```python
from build123d import *

# Parameters (mm, degrees)
EXTRUDE_1_DEPTH             = 8
CUT_EXTRUDE_1_DEPTH         = 5
HOLE_WIZARD_M51_D           = 5.2
HOLE_WIZARD_M51_DEPTH       = 4.2
HOLE_WIZARD_M51_CBORE_D     = 12
HOLE_WIZARD_M51_CBORE_DEPTH = 3
FILLET_1_R                  = 1


with BuildPart() as part:
    # Эскиз1 → Бобышка-Вытянуть1 (new body, symmetric)
    with BuildSketch(Plane.XY):
        Polygon((11, 0), (-11, 0), (-11, 9.2), (-6.75, 9.2), (-6.75, 5.7), (-5.25, 4.2), (5.25, 4.2), (6.75, 5.7), (6.75, 9.2), (11, 9.2), align=None)
    extrude(amount=EXTRUDE_1_DEPTH, both=True)

    # Эскиз2 → Вырез-Вытянуть1 (cut, symmetric)
    with BuildSketch(Plane.XY):
        Polygon((-11, 7.7), (-6.75, 7.7), (-6.75, 5.7), (-5.25, 4.2), (-6.5, 4.2), (-6.5, 0), (-11, 0), align=None)
    cut_extrude_1 = extrude(amount=CUT_EXTRUDE_1_DEPTH, both=True, mode=Mode.SUBTRACT)

    # Зеркальное отражение1: Вырез-Вытянуть1 across plane
    add(cut_extrude_1.mirror(Plane(origin=(0, 0, 0), x_dir=(0, 0, 1), z_dir=(1, 0, 0))), mode=Mode.SUBTRACT)

    # Цековка для  болта с шестигранной головкой M51
    with Locations(Plane(origin=(0, 4.2, 0), x_dir=(1, 0, 0), z_dir=(0, 1, 0))):
        with Locations((0, 0)):
            CounterBoreHole(HOLE_WIZARD_M51_D / 2, HOLE_WIZARD_M51_CBORE_D / 2, HOLE_WIZARD_M51_CBORE_DEPTH, depth=HOLE_WIZARD_M51_DEPTH)

    # Скругление1
    fillet_1_edges = [part.edges().sort_by_distance(p)[0] for p in [
        (11, 4.6, 8),
        (11, 4.6, -8),
        (-11, 4.6, -8),
        (-11, 4.6, 8),
    ]]
    fillet(fillet_1_edges, radius=FILLET_1_R)


solid = part.part
```
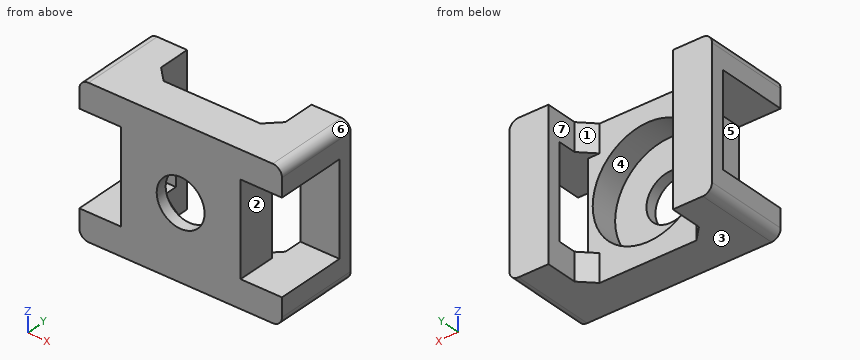
The listing builds one solid part. Answer for the finished solid, in the listing's coordinates (mm). Face numbers are marked on the shaded views. A direction names the side the tool comes from. Round coordinates to 2 decimals unless told otherwise and drop trailing zeros. Order: outer loops, then holes, each group sorted by start corner. A loop starts at its lowest first (then second) coordinate and runs counter-clockwise, first axis right, second up. Notation, with made-up numbers: (46, 57.25) - (88, 57.25) arc R7 cw to (88, 62.25) - close; hole circle Ø8 at (-12, -27.75). An arc over 180 degrees is marked (long way). Put each result on its own line as item: value. Start each with the question number.
(1) Given P1, Ø6, axis at x = 0, z = 0, coming from the +Y side; P2, Ø4, axis at x = -2, z = 3.5, coming from the +Y side; P3, Ø4.5, axis at y = 2, z = 2, coming from the -X side, each flat-ended and moving along its own axis, determine where each tip first touches the part or whether it passes through.
(2) Determine the mould class of the marked faces 1, 2 and 3 for opening direction X: released by +X, released by -X, zero draft, split by the parting line, or undercut.
(3) Find section D-D (y = 6.5). Give the vertices of the cut face in (x, z).
(4) Find section A-A (z = 0). Give the vertices of the cut face in (x, y).
(5) Find section B-B (y = 1.75). Give the vertices of the cut face in (x, z).
(6) Straight lines are drawn through the part: probe 1 along Z at (x, y) = (0, 0.3); probe 2 along Z at (x, y) = (0, 2.55); probe 3 along Y at (x, z) = (1.25, -3). For each, find the intervals that lie inside material, in ascending order. Write a range as from..to.
(7) For the marked faces 4, 5, 6 and 7, determine the directions among +Z, -Z, +X, -X, +Y, -Y from which every point of the face is accessible in a straight line to the end or side of a thin tool.
(8) Find section C-C (x = 0). Give the vertices of the cut face in (y, z).
Reply:
1. P1: y = 1.2
1. P2: y = 4.2
1. P3: x = -6.5
2. face 1: undercut
2. face 2: released by +X
2. face 3: zero draft
3. outline: (-11, -7) arc R1 ccw to (-10, -8) - (-6.75, -8) - (-6.75, -5) - (-11, -5) - close; (-11, 5) - (-6.75, 5) - (-6.75, 8) - (-10, 8) arc R1 ccw to (-11, 7) - close; (6.75, -8) - (10, -8) arc R1 ccw to (11, -7) - (11, -5) - (6.75, -5) - close; (6.75, 5) - (11, 5) - (11, 7) arc R1 ccw to (10, 8) - (6.75, 8) - close
4. outline: (-11, 7.7) - (-6.75, 7.7) - (-6.75, 9.2) - (-11, 9.2) - close; (-6.5, 0) - (-2.6, 0) - (-2.6, 1.2) - (-6, 1.2) - (-6, 4.2) - (-6.5, 4.2) - close; (2.6, 0) - (6.5, 0) - (6.5, 4.2) - (6, 4.2) - (6, 1.2) - (2.6, 1.2) - close; (6.75, 7.7) - (11, 7.7) - (11, 9.2) - (6.75, 9.2) - close
5. outline: (-11, -7) arc R1 ccw to (-10, -8) - (10, -8) arc R1 ccw to (11, -7) - (11, -5) - (6.5, -5) - (6.5, 5) - (11, 5) - (11, 7) arc R1 ccw to (10, 8) - (-10, 8) arc R1 ccw to (-11, 7) - (-11, 5) - (-6.5, 5) - (-6.5, -5) - (-11, -5) - close; hole circle Ø12 at (0, 0)
6. probe 1: -8..-2.6, 2.6..8
6. probe 2: -8..-6, 6..8
6. probe 3: 0..1.2
7. face 4: +Y
7. face 5: -X, +Y, -Y
7. face 6: +Z, +X, +Y, -Y
7. face 7: +Z, -Z, +Y
8. outline: (0, -8) - (4.2, -8) - (4.2, -6) - (1.2, -6) - (1.2, -2.6) - (0, -2.6) - close; (0, 2.6) - (1.2, 2.6) - (1.2, 6) - (4.2, 6) - (4.2, 8) - (0, 8) - close
